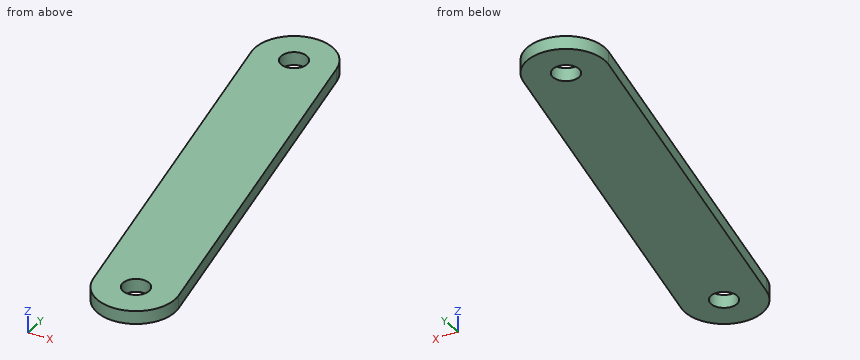
```python
from build123d import *

# Parameters (mm, degrees)
SKETCH_R  = 1
PAD_DEPTH = 1


with BuildPart() as part:
    # Sketch → Pad (new body)
    with BuildSketch(Plane.XY):
        with BuildLine():
            ThreePointArc((2.954423, 0.520945), (-0.520945, 2.954423), (-2.954423, -0.520945))
            Line((-2.954423, -0.520945), (2.255022, -30.065177))
            ThreePointArc((2.255022, -30.065177), (5.73039, -32.498656), (8.163869, -29.023288))
            Line((2.954423, 0.520945), (8.163869, -29.023288))
        make_face()
        Circle(SKETCH_R, mode=Mode.SUBTRACT)
        with Locations((5.209445, -29.544233)):
            Circle(SKETCH_R, mode=Mode.SUBTRACT)
    extrude(amount=PAD_DEPTH)


solid = part.part
```
Work out the finished part from the listing and answer in its coordinate system (mm). Give positions to 0.01 mm unless a question says otherwise; leave off trailing zeros. Loops run counter-clockwise (first coordinate to the right, second up) from the corner with the lowest first, then second, coordinate; pieces in that order, holes last. Notation, with made-up numbers: (47.5, -16) - (75.5, -16) arc R15 cw to (75.5, -3) - close; hole circle Ø2 at (59.25, 78). An arc over 180 degrees is marked (long way). Use CSV: the item, a comma, the result in double quotes. Start each with the question number.
(1) Find section D-D, the plane y = -6.5. Determine the outline of the cut face in (x, z), plus the area to 3 significant figures.
(2) Find the intervals of material crossed by L1, parallel to X at y = 0.5, z = 0.25; L2, parallel to X at y = -16, z = 0.8; L3, parallel to Y at x = 2.5, z = 0.5, in increasing order.
(3) This flat-tipped pin is pushed along its axis until it touches: pin 1 (5 mm diameter, centred on x = -1.5, y = -24.5, fed in from -Z). Where does it stop, or does it pass through?
(4) Find section B-B, the plane y = 0. Determine the outline of the cut face in (x, z).
(5) Find section A-A, the plane x = 5.5. Determine the outline of the cut face in (y, z).
Results found:
1,outline,"(-1.9, 0) - (4.19, 0) - (4.19, 1) - (-1.9, 1) - close"
1,area,"6.09 mm^2"
2,L1,"-2.96 to -0.87, 0.87 to 2.96"
2,L2,"-0.23 to 5.87"
2,L3,"-30.83 to 1.66"
3,pin 1,"through"
4,outline,"(-3, 0) - (-1, 0) - (-1, 1) - (-3, 1) - close; (1, 0) - (3.05, 0) - (3.05, 1) - (1, 1) - close"
5,outline,"(-32.53, 0) - (-30.5, 0) - (-30.5, 1) - (-32.53, 1) - close; (-28.59, 0) - (-13.92, 0) - (-13.92, 1) - (-28.59, 1) - close"
